Here's how the part is built. I have some questions about the finished solid (model axes, mm). A direction names the side the tool comes from. Round coordinates to 2 decimals unless told otherwise and drop trailing zeros. Order: outer loops, then holes, each group sorted by start corner. A loop starts at its lowest first (then second) coordinate and runs counter-clockwise, first axis right, second up. Notation, with made-up numbers: (82.5, 85.25) -> (115.5, 85.25) arc R36 ccw to (115.5, 123.25) -> close; hole circle Ø7 at (34.25, 88). An arc over 180 degrees is marked (long way). Use a Markdown table: item, result. Add a question column.
(1) If I drill on probe 1 along X at (y, z) = (-12, 31); probe 2 along Y at (x, z) = (-12, 6.5); probe 3 along X at (y, z) = (-22, 18), over which ranges is the centre line in solid material (lowest first)?
(2) I'm going to push flat-ended pins straight in: P1, Ø8, axis at x = 12, y = 32.5, coming from the -Z side; P2, Ø4, axis at x = -12.5, y = 23, coming from the -Z side; P3, Ø2, axis at x = 19.5, z = 25.5, coming from the +Y side; P4, Ø3, axis at x = 13, y = 32.5, coming from the -Z side. Where does each tip first touch, or does it pass through?
(3) I want a section at B-B, the plane y = -2. Please give me the cut outline in (x, z).
(4) Thinking about a two-plate mould opening in Z: for faces 4 (the face through (0, 1, 0)), 5 (the face through (-28, -19, 45.365)), 6 (the face through (0, -8.3, 5)), which applies, pulls with the +Z half, pulls with the -Z half, needs draft (parallel to the pull), parting line crosses it, or undercut?
(5) On a 3-axis mill with a long thin cutter (end or side, diameter ignored), from which of +Z, -Z, +X, -X, +Y, -Y can I reach the whole of each face in a straight line? I mean faces 1 (the face through (21.877, -18.794, 41.434)), 2 (the face through (7.23, 34, 2.46)), 3 (the face through (-11.586, 24.433, 9.042)). Say none if no direction works.
(6) I want a section at A-A, the plane x = 0. Please give me the cut outline in (y, z).
(7) I want a section at C-C, the plane z = 21. Give the number of separate pieces and of enclosed holes in the cut face, then the cut area to 3 significant figures.
from build123d import *

# Parameters (mm, degrees)
SKETCH1_W                      = 60
SKETCH1_H                      = 53
BOSS_EXTRUDE1_DEPTH            = 12
SKETCH2_W                      = 60
SKETCH2_H                      = 21
BOSS_EXTRUDE2_DEPTH            = 12
SKETCH4_W                      = 40.2
SKETCH4_H                      = 18.2
CUT_EXTRUDE1_DEPTH             = 10
SKETCH5_R                      = 1.9
CUT_EXTRUDE2_DEPTH             = 43.405777908
SKETCH8_W                      = 60
SKETCH8_H                      = 16.2
SKETCH8_R                      = 1.9
BOSS_EXTRUDE3_DEPTH            = 25
CUT_EXTRUDE3_DEPTH             = 15.2
FILLET1_R                      = 5
FILLET2_R                      = 7
BOSS_EXTRUDE5_REACH            = 80.166
CUT_EXTRUDE4_DEPTH             = 69.773832233
MIRROR1_START                  = -26.5
MIRROR1_DEPTH                  = 15.2
MIRROR1_START_2                = -11.3
MIRROR1_2_DEPTH                = 3
SKETCH10_W                     = 60
SKETCH10_H                     = 49
BOSS_EXTRUDE4_DEPTH            = 12
SKETCH16_W                     = 60
SKETCH16_H                     = 12
BOSS_EXTRUDE6_DEPTH            = 12
M5X0_8_TAPPED_HOLE1_D          = 4.2
CBORE_FOR_M3_SHCS1_D           = 3.4
CBORE_FOR_M3_SHCS1_CBORE_D     = 6.5
CBORE_FOR_M3_SHCS1_CBORE_DEPTH = 6
CBORE_FOR_M5_SHCS1_D           = 5.5
CBORE_FOR_M5_SHCS1_CBORE_D     = 10
CBORE_FOR_M5_SHCS1_CBORE_DEPTH = 5


# Read off the part's stored shape, not the designer's step: Mirror1
with BuildPart() as part:
    # Sketch1 → Boss-Extrude1 (new body)
    with BuildSketch(Plane.XY):
        Rectangle(SKETCH1_W, SKETCH1_H)
    extrude(amount=BOSS_EXTRUDE1_DEPTH)

    # Sketch2 → Boss-Extrude2 (add)
    with BuildSketch(Plane(origin=(0, 0, 12), x_dir=(-1, 0, 0), z_dir=(0, 0, -1))):
        with Locations((0, -16)):
            Rectangle(SKETCH2_W, SKETCH2_H)
    extrude(amount=-BOSS_EXTRUDE2_DEPTH)

    # Sketch4 → Cut-Extrude1 (cut)
    with BuildSketch(Plane(origin=(0, 0, 0), x_dir=(-1, 0, 0), z_dir=(0, 0, -1))):
        with Locations((0, -17.4)):
            Rectangle(SKETCH4_W, SKETCH4_H)
    extrude(amount=-CUT_EXTRUDE1_DEPTH, mode=Mode.SUBTRACT)

    # Sketch5 → Cut-Extrude2 (cut, through all)
    with BuildSketch(Plane(origin=(0, 0, 10), x_dir=(-1, 0, 0), z_dir=(0, 0, -1))):
        with Locations((0, -12.8)):
            Circle(SKETCH5_R)
        with Locations((0, -22)):
            Circle(SKETCH5_R)
    extrude(amount=-CUT_EXTRUDE2_DEPTH, mode=Mode.SUBTRACT)

    # Sketch8 → Boss-Extrude3 (add)
    with BuildSketch(Plane.XY.offset(24)):
        with Locations((0, -18.4)):
            Rectangle(SKETCH8_W, SKETCH8_H)
        with Locations(Location((0, -22, 0), (0, 0, 180))):
            Circle(SKETCH8_R, mode=Mode.SUBTRACT)
        with Locations(Location((0, -12.8, 0), (0, 0, 180))):
            Circle(SKETCH8_R, mode=Mode.SUBTRACT)
    extrude(amount=BOSS_EXTRUDE3_DEPTH)

    # Sketch9 → Cut-Extrude3 (cut)
    with BuildSketch(Plane.XZ.offset(26.5)):
        Polygon((20.1, 10), (25.1, 10), (17.051847549, 45.365), (30, 45.365), (30, 43.365), (19.558131605, 43.365), (22, 32.635), (30, 32.635), (30, 30.635), (22.455147884, 30.635), (27.606284055, 8), (20.1, 8), align=None)
    extrude(amount=-CUT_EXTRUDE3_DEPTH, mode=Mode.SUBTRACT)

    # Fillet1
    fillet1_edges = [part.edges().sort_by_distance(p)[0] for p in [
        (19.558131605, -18.9, 43.365),
        (22.455147884, -18.9, 30.635),
        (25.1, -18.9, 10),
    ]]
    fillet(fillet1_edges, radius=FILLET1_R)

    # Fillet2
    # the kernel refuses this fillet: 7 mm, written as the material it adds along each edge
    with BuildSketch(Plane(origin=(27.606284055, -26.5, 8), x_dir=(-1, 0, 0), z_dir=(0, 1, 0))) as fillet2_piece_1:
        with BuildLine():
            CenterArc((8.746780519, 6.889206669), FILLET2_R, 167.179324342, 92.613163385)
            Line((1.921295117, 8.442509286), (1.784785409, 8.473575339))
            Line((1.784785409, 8.473575339), (-0.136509708, 0.031066052))
            Line((-0.136509708, 0.031066052), (0, -0.14))
            ThreePointArc((0, -0.14), (3.753142028, -0.14), (7.481474126, -0.137784133))
            Line((7.481474126, -0.137784133), (7.506284055, 0))
        make_face()
    extrude(amount=15.2)
    with BuildSketch(Plane(origin=(17.051847549, -26.5, 45.365), x_dir=(0.22190037393070375, 0, -0.9750693432004792), z_dir=(0, 1, 0))) as fillet2_piece_2:
        with BuildLine():
            CenterArc((FILLET2_R * 1.25314202775, -FILLET2_R), FILLET2_R, 90, 102.820675658)
            Line((FILLET2_R * 0.278072684545, -FILLET2_R * 1.22190037393), (FILLET2_R * 0.258571297681, -FILLET2_R * 1.22633838141))
            Line((FILLET2_R * 0.258571297681, -FILLET2_R * 1.22633838141), (-FILLET2_R * 0.0250628405549, FILLET2_R * 0.02))
            Line((-FILLET2_R * 0.0250628405549, FILLET2_R * 0.02), (FILLET2_R * 1.25314202775, FILLET2_R * 0.02))
            Line((FILLET2_R * 1.25314202775, FILLET2_R * 0.02), (FILLET2_R * 1.25314202775, 0))
        make_face()
    extrude(amount=15.2)

    # Sketch14 → Boss-Extrude5 (add, up to next)
    with BuildSketch(Plane.XZ.offset(26.5), mode=Mode.PRIVATE) as boss_extrude5_sk1:
        with BuildLine():
            Line((22, 32.635), (22.758425927, 29.30234284))
            ThreePointArc((22.758425927, 29.30234284), (25.30555422, 31.745294587), (28.720858022, 32.635))
            Line((28.720858022, 32.635), (22, 32.635))
        make_face()
    boss_extrude5_tool1 = extrude(boss_extrude5_sk1.sketch, amount=-BOSS_EXTRUDE5_REACH, mode=Mode.PRIVATE) - part.part
    add(boss_extrude5_tool1.solids().sort_by_distance((23.8726, -26.5, 31.664798))[0])

    # Sketch15 → Cut-Extrude4 (cut, through all)
    with BuildSketch(Plane.XZ.offset(11.3)):
        with BuildLine():
            Line((25.684988939, 16.442509286), (23.709636577, 16.10950187))
            ThreePointArc((23.709636577, 16.10950187), (23.108491418, 12.40554417), (20.1, 10.16285437))
            Line((20.1, 10.16285437), (20.1, 0))
            Line((20.1, 0), (25.859503536, 0))
            Line((25.859503536, 0), (25.859503536, 14.889206669))
            ThreePointArc((25.859503536, 14.889206669), (25.815738072, 15.670744314), (25.684988939, 16.442509286))
        make_face()
    extrude(amount=CUT_EXTRUDE4_DEPTH, mode=Mode.SUBTRACT)

    # Mirror1 outline → Mirror1 (cut)
    with BuildSketch(Plane(origin=(0, 0, 0), x_dir=(1, 0, 0), z_dir=(0, 1, 0)).offset(MIRROR1_START)):
        with BuildLine():
            Line((-30, -32.635), (-28.720858022, -32.635))
            ThreePointArc((-28.720858022, -32.635), (-25.30555422, -31.745294587), (-22.758425927, -29.30234284))
            Line((-22.758425927, -29.30234284), (-20.948495028, -37.25549813))
            ThreePointArc((-20.948495028, -37.25549813), (-21.915676615, -41.483692887), (-25.823841744, -43.365))
            Line((-25.823841744, -43.365), (-30, -43.365))
            Line((-30, -43.365), (-30, -45.365))
            Line((-30, -45.365), (-25.823841744, -45.365))
            ThreePointArc((-25.823841744, -45.365), (-20.352410563, -42.731170042), (-18.998356341, -36.811697382))
            Line((-18.998356341, -36.811697382), (-23.709636577, -16.10950187))
            ThreePointArc((-23.709636577, -16.10950187), (-22.74245499, -11.881307113), (-18.834289861, -10))
            Line((-18.834289861, -10), (-20.1, -10))
            Line((-20.1, -10), (-20.1, 0))
            Line((-20.1, 0), (-25.859503536, 0))
            Line((-25.859503536, 0), (-25.859503536, -14.889206669))
            ThreePointArc((-25.859503536, -14.889206669), (-25.815738072, -15.670744314), (-25.684988939, -16.442509286))
            Line((-25.684988939, -16.442509286), (-23.845511306, -24.52549813))
            ThreePointArc((-23.845511306, -24.52549813), (-24.812692893, -28.753692887), (-28.720858022, -30.635))
            Line((-28.720858022, -30.635), (-30, -30.635))
            Line((-30, -30.635), (-30, -32.635))
        make_face()
    extrude(amount=MIRROR1_DEPTH, mode=Mode.SUBTRACT)

    # Mirror1 2 outline → Mirror1 2 (cut)
    with BuildSketch(Plane(origin=(0, 0, 0), x_dir=(1, 0, 0), z_dir=(0, 1, 0)).offset(MIRROR1_START_2)):
        with BuildLine():
            Line((-18.834289861, -10), (-20.1, -10))
            Line((-20.1, -10), (-20.1, -10.16285437))
            ThreePointArc((-20.1, -10.16285437), (-19.472361899, -10.040880716), (-18.834289861, -10))
        make_face()
    extrude(amount=MIRROR1_2_DEPTH, mode=Mode.SUBTRACT)

    # Sketch10 → Boss-Extrude4 (add)
    with BuildSketch(Plane.XZ.offset(26.5)):
        with Locations((0, 24.5)):
            Rectangle(SKETCH10_W, SKETCH10_H)
    extrude(amount=BOSS_EXTRUDE4_DEPTH)

    # Sketch16 → Boss-Extrude6 (add)
    with BuildSketch(Plane.XY.offset(12)):
        with Locations((0, 32.5)):
            Rectangle(SKETCH16_W, SKETCH16_H)
    extrude(amount=-BOSS_EXTRUDE6_DEPTH)

    # M5x0.8 Tapped Hole1 (through all)
    with Locations(Plane(origin=(0, 0, 0), x_dir=(-1, 0, 0), z_dir=(0, 0, -1))):
        with Locations((-24, 32.5), (-24, -32.5), (24, -32.5), (24, 32.5), (-12, -32.5), (12, -32.5)):
            Hole(M5X0_8_TAPPED_HOLE1_D / 2)

    # CBORE for M3 SHCS1 (through all)
    with Locations(Plane(origin=(0, 0, 0), x_dir=(-1, 0, 0), z_dir=(0, 0, -1))):
        with Locations((12.5, -2), (-12.5, -2), (-12.5, 23), (12.5, 23)):
            CounterBoreHole(CBORE_FOR_M3_SHCS1_D / 2, CBORE_FOR_M3_SHCS1_CBORE_D / 2, CBORE_FOR_M3_SHCS1_CBORE_DEPTH)

    # CBORE for M5 SHCS1 (through all)
    with Locations(Plane(origin=(0, 0, 0), x_dir=(-1, 0, 0), z_dir=(0, 0, -1))):
        with Locations((-12, 32.5), (12, 32.5)):
            CounterBoreHole(CBORE_FOR_M5_SHCS1_D / 2, CBORE_FOR_M5_SHCS1_CBORE_D / 2, CBORE_FOR_M5_SHCS1_CBORE_DEPTH)


solid = part.part
Taken from the geometry:
| question | item | result |
|---|---|---|
| 1 | probe 1 | x = -24.22 to -22.37, -20.32 to -1.72, 1.72 to 20.32, 22.37 to 24.22 |
| 1 | probe 2 | y = -38.5 to -34.6, -30.4 to -26.5, -8.3 to -3.62, -0.38 to 21.38, 24.62 to 29.75, 35.25 to 38.5 |
| 1 | probe 3 | x = -30 to -25.33, -23.28 to -1.9, 1.9 to 23.28, 25.33 to 30 |
| 2 | P1 | stops at z = 5 |
| 2 | P2 | stops at z = 6 |
| 2 | P3 | stops at y = -10.3 |
| 2 | P4 | passes through |
| 3 | outline | (-30, 0) -> (-15.75, 0) -> (-15.75, 6) -> (-14.2, 6) -> (-14.2, 12) -> (-30, 12) -> close; (-10.8, 6) -> (-9.25, 6) -> (-9.25, 0) -> (9.25, 0) -> (9.25, 6) -> (10.8, 6) -> (10.8, 12) -> (-10.8, 12) -> close; (14.2, 6) -> (15.75, 6) -> (15.75, 0) -> (30, 0) -> (30, 12) -> (14.2, 12) -> close |
| 4 | face 4 | pulls with the -Z half |
| 4 | face 5 | undercut |
| 4 | face 6 | needs draft |
| 5 | face 1 | none |
| 5 | face 2 | -Z |
| 5 | face 3 | +Z, -Z |
| 6 | outline | (-38.5, 0) -> (-26.5, 0) -> (-26.5, 10) -> (-23.9, 10) -> (-23.9, 49) -> (-38.5, 49) -> close; (-20.1, 10) -> (-14.7, 10) -> (-14.7, 49) -> (-20.1, 49) -> close; (-10.9, 10) -> (-8.3, 10) -> (-8.3, 0) -> (38.5, 0) -> (38.5, 12) -> (-5.5, 12) -> (-5.5, 24) -> (-10.3, 24) -> (-10.3, 49) -> (-10.9, 49) -> close |
| 7 | separate pieces | 1 |
| 7 | enclosed holes | 8 |
| 7 | area | 1,840 mm2 |
